Design review of the part built by this model. Coordinates are the model's own, in mm. A direction names the side the tool comes from. Coordinates: 2 decimals unless noted, no trailing zeros. Write each loop counter-clockwise with the first axis right and the second up, starting at its lowest first coordinate (ties: lowest second). Pieces come first, ordered by that corner, then holes. Notation, with made-up numbers: (38.25, 59) - (79.25, 59) arc R22 cw to (79.25, 83) - close; hole circle Ø11 at (-23.75, 66). An arc over 180 degrees is marked (long way). One line per item, written item: value.
from build123d import *

# Parameters (mm, degrees)
F1_DEPTH = 1.5
F0_R     = 1.1
F2_DEPTH = 1.5
F3_DEPTH = 2.3
F0_R_2   = 4.25
F4_DEPTH = 0.9


with BuildPart() as f1:
    # F0 (on Front) → F1 (new body)
    with BuildSketch(Plane.XZ):
        with BuildLine():
            Line((-4.7360679775, 12.5), (-12, 12.5))
            Line((-12, 12.5), (-12, 0))
            ThreePointArc((-12, 0), (-10.101019661, 5.6986401986), (-5.1632631341, 9.119047619))
            ThreePointArc((-5.1632631341, 9.119047619), (-5.476335177, 10.8760703579), (-4.7360679775, 12.5))
        make_face()
    extrude(amount=F1_DEPTH)



with BuildPart() as f1b:
    # F0 (on Front) → F1, piece 2 (new body)
    with BuildSketch(Plane.XZ):
        with BuildLine():
            ThreePointArc((-5.1632631341, -9.119047619), (-10.101019661, -5.6986401986), (-12, 0))
            Line((-12, 0), (-12, -12.5))
            Line((-12, -12.5), (-4.7360679775, -12.5))
            ThreePointArc((-4.7360679775, -12.5), (-5.476335177, -10.8760703579), (-5.1632631341, -9.119047619))
        make_face()
    extrude(amount=F1_DEPTH)


with BuildPart() as f1c:
    # F0 (on Front) → F1, piece 3 (new body)
    with BuildSketch(Plane.XZ):
        with BuildLine():
            Line((12, 12.5), (-0.2639320225, 12.5))
            ThreePointArc((-0.2639320225, 12.5), (0.3025170769, 11.5704662693), (0.5, 10.5))
            ThreePointArc((0.5, 10.5), (0.4146002644, 9.7892923957), (0.1632631341, 9.119047619))
            ThreePointArc((0.1632631341, 9.119047619), (5.101019661, 5.6986401986), (7, 0))
            ThreePointArc((7, 0), (5.101019661, -5.6986401986), (0.1632631341, -9.119047619))
            ThreePointArc((0.1632631341, -9.119047619), (0.4146002644, -9.7892923957), (0.5, -10.5))
            ThreePointArc((0.5, -10.5), (0.3025170769, -11.5704662693), (-0.2639320225, -12.5))
            Line((-0.2639320225, -12.5), (12, -12.5))
            Line((12, -12.5), (12, 12.5))
        make_face()
        with Locations((10, -10.5)):
            Circle(F0_R, mode=Mode.SUBTRACT)
        with Locations((10, 10.5)):
            Circle(F0_R, mode=Mode.SUBTRACT)
    extrude(amount=F1_DEPTH)


with BuildPart() as f1d:
    # F0 (on Front) → F1, piece 4 (new body)
    with BuildSketch(Plane.XZ):
        with BuildLine():
            ThreePointArc((-2.9357751714, 9.49), (-4.0605803478, 9.370943868), (-5.1632631341, 9.119047619))
            ThreePointArc((-5.1632631341, 9.119047619), (-4.956519224, 8.7779334211), (-4.7063489833, 8.4672619048))
            ThreePointArc((-4.7063489833, 8.4672619048), (-2.5, 8.75), (-0.2936510167, 8.4672619048))
            ThreePointArc((-0.2936510167, 8.4672619048), (-0.043480776, 8.7779334211), (0.1632631341, 9.119047619))
            ThreePointArc((0.1632631341, 9.119047619), (-0.9394196522, 9.370943868), (-2.0642248286, 9.49))
            ThreePointArc((-2.0642248286, 9.49), (-2.5, 9.4), (-2.9357751714, 9.49))
        make_face()
    extrude(amount=F1_DEPTH)


with BuildPart() as f1_1:
    add(f1.part)

    add(f1b.part)  # F2 merges F1b

    add(f1c.part)  # F2 merges F1c

    add(f1d.part)  # F2 merges F1d
    # F0 (on Front) → F2 (join)
    with BuildSketch(Plane.XZ):
        with BuildLine():
            Line((12, 12.5), (-0.2639320225, 12.5))
            ThreePointArc((-0.2639320225, 12.5), (0.3025170769, 11.5704662693), (0.5, 10.5))
            ThreePointArc((0.5, 10.5), (0.4146002644, 9.7892923957), (0.1632631341, 9.119047619))
            ThreePointArc((0.1632631341, 9.119047619), (5.101019661, 5.6986401986), (7, 0))
            ThreePointArc((7, 0), (5.101019661, -5.6986401986), (0.1632631341, -9.119047619))
            ThreePointArc((0.1632631341, -9.119047619), (0.4146002644, -9.7892923957), (0.5, -10.5))
            ThreePointArc((0.5, -10.5), (0.3025170769, -11.5704662693), (-0.2639320225, -12.5))
            Line((-0.2639320225, -12.5), (12, -12.5))
            Line((12, -12.5), (12, 12.5))
        make_face()
        with Locations((10, -10.5)):
            Circle(F0_R, mode=Mode.SUBTRACT)
        with Locations((10, 10.5)):
            Circle(F0_R, mode=Mode.SUBTRACT)
        with BuildLine():
            ThreePointArc((-2.9357751714, -9.49), (-4.0605803478, -9.370943868), (-5.1632631341, -9.119047619))
            ThreePointArc((-5.1632631341, -9.119047619), (-5.476335177, -10.8760703579), (-4.7360679775, -12.5))
            Line((-4.7360679775, -12.5), (-0.2639320225, -12.5))
            ThreePointArc((-0.2639320225, -12.5), (0.3025170769, -11.5704662693), (0.5, -10.5))
            ThreePointArc((0.5, -10.5), (0.4146002644, -9.7892923957), (0.1632631341, -9.119047619))
            ThreePointArc((0.1632631341, -9.119047619), (-0.9394196522, -9.370943868), (-2.0642248286, -9.49))
            ThreePointArc((-2.0642248286, -9.49), (-1.5809372468, -9.8955799013), (-1.4, -10.5))
            ThreePointArc((-1.4, -10.5), (-3.1044200987, -11.4190627532), (-2.9357751714, -9.49))
        make_face()
        with BuildLine():
            Line((-0.2639320225, 12.5), (-4.7360679775, 12.5))
            ThreePointArc((-4.7360679775, 12.5), (-5.476335177, 10.8760703579), (-5.1632631341, 9.119047619))
            ThreePointArc((-5.1632631341, 9.119047619), (-4.0605803478, 9.370943868), (-2.9357751714, 9.49))
            ThreePointArc((-2.9357751714, 9.49), (-3.1044200987, 11.4190627532), (-1.4, 10.5))
            ThreePointArc((-1.4, 10.5), (-1.5809372468, 9.8955799013), (-2.0642248286, 9.49))
            ThreePointArc((-2.0642248286, 9.49), (-0.9394196522, 9.370943868), (0.1632631341, 9.119047619))
            ThreePointArc((0.1632631341, 9.119047619), (0.4146002644, 9.7892923957), (0.5, 10.5))
            ThreePointArc((0.5, 10.5), (0.3025170769, 11.5704662693), (-0.2639320225, 12.5))
        make_face()
        with BuildLine():
            ThreePointArc((-4.7063489833, -8.4672619048), (-4.956519224, -8.7779334211), (-5.1632631341, -9.119047619))
            ThreePointArc((-5.1632631341, -9.119047619), (-4.0605803478, -9.370943868), (-2.9357751714, -9.49))
            ThreePointArc((-2.9357751714, -9.49), (-2.5, -9.4), (-2.0642248286, -9.49))
            ThreePointArc((-2.0642248286, -9.49), (-0.9394196522, -9.370943868), (0.1632631341, -9.119047619))
            ThreePointArc((0.1632631341, -9.119047619), (-0.043480776, -8.7779334211), (-0.2936510167, -8.4672619048))
            ThreePointArc((-0.2936510167, -8.4672619048), (-2.5, -8.75), (-4.7063489833, -8.4672619048))
        make_face()
    extrude(amount=F2_DEPTH)

    # F0 (on Front) → F3 (join)
    with BuildSketch(Plane.XZ):
        with BuildLine():
            ThreePointArc((-5.1632631341, 9.119047619), (-10.101019661, 5.6986401986), (-12, 0))
            ThreePointArc((-12, 0), (-10.101019661, -5.6986401986), (-5.1632631341, -9.119047619))
            ThreePointArc((-5.1632631341, -9.119047619), (-4.956519224, -8.7779334211), (-4.7063489833, -8.4672619048))
            ThreePointArc((-4.7063489833, -8.4672619048), (-11.25, 0), (-4.7063489833, 8.4672619048))
            ThreePointArc((-4.7063489833, 8.4672619048), (-4.956519224, 8.7779334211), (-5.1632631341, 9.119047619))
        make_face()
        with BuildLine():
            ThreePointArc((7, 0), (5.101019661, 5.6986401986), (0.1632631341, 9.119047619))
            ThreePointArc((0.1632631341, 9.119047619), (-0.043480776, 8.7779334211), (-0.2936510167, 8.4672619048))
            ThreePointArc((-0.2936510167, 8.4672619048), (4.4234403877, 5.3505582137), (6.25, 0))
            ThreePointArc((6.25, 0), (4.4234403877, -5.3505582137), (-0.2936510167, -8.4672619048))
            ThreePointArc((-0.2936510167, -8.4672619048), (-0.043480776, -8.7779334211), (0.1632631341, -9.119047619))
            ThreePointArc((0.1632631341, -9.119047619), (5.101019661, -5.6986401986), (7, 0))
        make_face()
    extrude(amount=F3_DEPTH)

    # F0 (on Front) → F4 (join)
    with BuildSketch(Plane.XZ):
        with BuildLine():
            ThreePointArc((-0.2936510167, 8.4672619048), (-2.5, 7.5), (-4.7063489833, 8.4672619048))
            ThreePointArc((-4.7063489833, 8.4672619048), (-11.25, 0), (-4.7063489833, -8.4672619048))
            ThreePointArc((-4.7063489833, -8.4672619048), (-2.5, -7.5), (-0.2936510167, -8.4672619048))
            ThreePointArc((-0.2936510167, -8.4672619048), (4.4234403877, -5.3505582137), (6.25, 0))
            ThreePointArc((6.25, 0), (4.4234403877, 5.3505582137), (-0.2936510167, 8.4672619048))
        make_face()
        with Locations((-2.5, 0)):
            Circle(F0_R_2, mode=Mode.SUBTRACT)
        with BuildLine():
            ThreePointArc((-0.2936510167, 8.4672619048), (-2.5, 8.75), (-4.7063489833, 8.4672619048))
            ThreePointArc((-4.7063489833, 8.4672619048), (-2.5, 7.5), (-0.2936510167, 8.4672619048))
        make_face()
        with BuildLine():
            ThreePointArc((-0.2936510167, -8.4672619048), (-2.5, -7.5), (-4.7063489833, -8.4672619048))
            ThreePointArc((-4.7063489833, -8.4672619048), (-2.5, -8.75), (-0.2936510167, -8.4672619048))
        make_face()
    extrude(amount=F4_DEPTH)


solid = f1_1.part
1. Insertion check: pin 1 Ø2 at (x, z) = (-2.5, -10.5) entering from +Y; pin 2 Ø14 at (x, z) = (-2, -1) entering from -Y; pin 3 Ø3 at (x, z) = (10, -10.5) entering from -Y. Each pin has a flat end and moves straight along its axis. Give the tip position at first contact, or say it passes through.
Answer block:
pin 1: passes through
pin 2: stops at y = -0.9
pin 3: stops at y = -1.5
2. Wall thickness on line 1 along Z through (x, y) = (10, -1); line 2 along Z through (x, y) = (-2.5, -0.85); line 3 along X through (y, z) = (-0.45, -10.25): over which ranges is each line inside the solid? List them lowest first.
Answer block:
line 1: z = -12.5 to -11.6, -9.4 to 9.4, 11.6 to 12.5
line 2: z = -12.5 to -11.6, -9.4 to -4.25, 4.25 to 9.4, 11.6 to 12.5
line 3: x = -12 to -3.57, -1.43 to 8.93, 11.07 to 12
3. Mouldability with a two-part tool opening along X and no side actions: class faces 3 (the face through (0, -1, -12.5)), 4 (the face through (-12, -1, 0)), 5 (the face through (11.016, -0.74, 10.079)), 6 (the face through (-5, -0.9, -4)) as released by +X, released by -X, zero draft, split by the parting line, or undercut.
Answer block:
face 3: zero draft
face 4: released by -X
face 5: undercut
face 6: undercut
4. Consider section D-D, the plane z = 10. Write out the cut boundary in (x, y).
Answer block:
outline: (-12, -1.5) - (-3.48, -1.5) - (-3.48, 0) - (-12, 0) - close; (-1.52, -1.5) - (9.02, -1.5) - (9.02, 0) - (-1.52, 0) - close; (10.98, -1.5) - (12, -1.5) - (12, 0) - (10.98, 0) - close
5. Consider section B-B, the plane y = -0.4. Write out the cut boundary in (x, z).
Answer block:
outline: (-12, -12.5) - (12, -12.5) - (12, 12.5) - (-12, 12.5) - close; hole circle Ø8.5 at (-2.5, 0); hole circle Ø2.2 at (-2.5, -10.5); hole circle Ø2.2 at (-2.5, 10.5); hole circle Ø2.2 at (10, -10.5); hole circle Ø2.2 at (10, 10.5)
6. Consider section C-C, the plane x = -2.5. Write out the cut boundary in (y, z), then the cut area to 4 significant figures.
Answer block:
outline: (-1.5, -12.5) - (0, -12.5) - (0, -11.6) - (-1.5, -11.6) - close; (-1.5, -9.4) - (0, -9.4) - (0, -4.25) - (-0.9, -4.25) - (-0.9, -8.75) - (-1.5, -8.75) - close; (-1.5, 8.75) - (-0.9, 8.75) - (-0.9, 4.25) - (0, 4.25) - (0, 9.4) - (-1.5, 9.4) - close; (-1.5, 11.6) - (0, 11.6) - (0, 12.5) - (-1.5, 12.5) - close
area: 12.75 mm^2
7. For faces 1 (the face through (0, -1, 12.5)), 2 (the face through (8, -1.5, 0)), list the 3-axis set-ups (+Z, -Z, +X, -X, +Y, -Y) from which the entire face can be reached by the end or side of a thin tool; tool diameter is ignored.
Answer block:
face 1: +Z, +X, -X, +Y, -Y
face 2: -Y
8. Consider section A-A, the plane x = 10. Write out the cut boundary in (y, z).
Answer block:
outline: (-1.5, -12.5) - (0, -12.5) - (0, -11.6) - (-1.5, -11.6) - close; (-1.5, -9.4) - (0, -9.4) - (0, 9.4) - (-1.5, 9.4) - close; (-1.5, 11.6) - (0, 11.6) - (0, 12.5) - (-1.5, 12.5) - close
